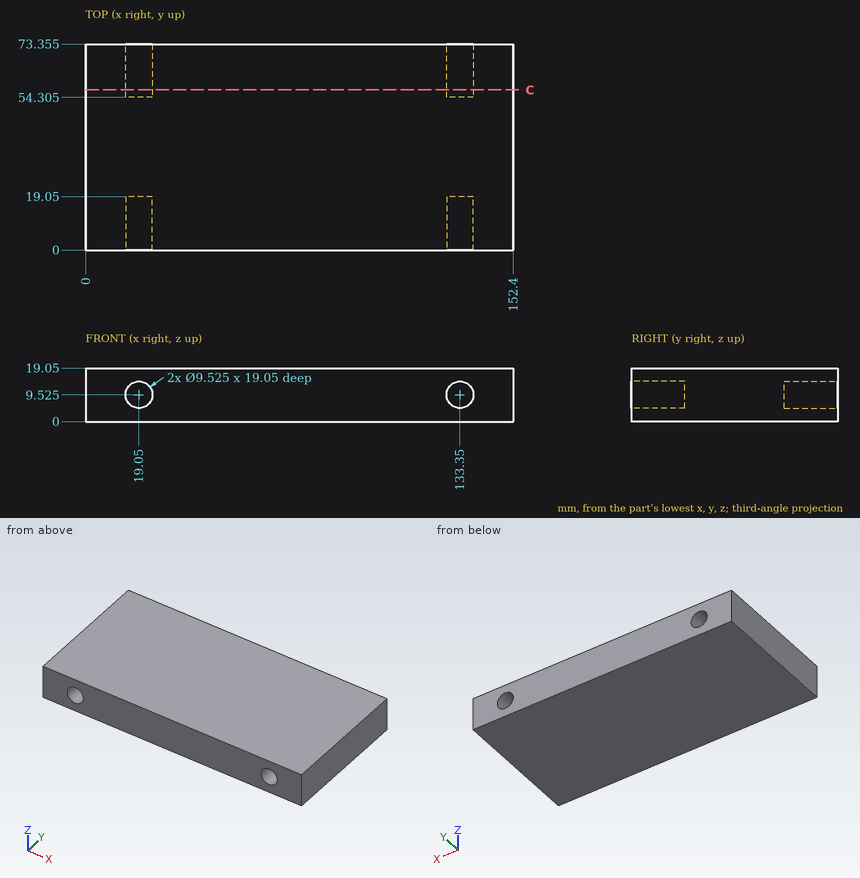
Input: dimensioned drawing with shaded views. Units: mm. Origin: part minimum x, y, z. Round coordinates to 2 decimals unless told otherwise and drop trailing zeros. One line per item, written item: value. Start each with the question number.
Q1. Pin query (flat end, axial travel): pin 1 (7.5 mm diameter, centred on x = 17.5, z = 8, fed in from -Y); pin 2 (3 mm diameter, centred on x = 17, z = 9.5, fed in from +Y) (3 decimals); pin 3 (8.5 mm diameter, centred on x = 19.05, z = 9.525, fed in from -Y). Return the tip coordinate at first contact, or that it passes through.
Q2. Material intervals for probe 1 along X at (y, z) = (67, 9); probe 2 along X at (y, z) = (6.5, 11.25); probe 3 along Z at (x, y) = (19.05, 8.25), sorted ascending.
Q3. Section query C-C (y = 57). Give the number of separate pieces and of enclosed holes in the cut face, plus the area to 3 significant figures.
Findings below:
1. pin 1: y = 0
1. pin 2: y = 54.305
1. pin 3: y = 19.05
2. probe 1: 0 to 14.32, 23.78 to 128.62, 138.08 to 152.4
2. probe 2: 0 to 14.61, 23.49 to 128.91, 137.79 to 152.4
2. probe 3: 0 to 4.76, 14.29 to 19.05
3. separate pieces: 1
3. enclosed holes: 2
3. area: 2,760 mm²
